Can you work these out from the model? Positions are in its coordinate system, mm. Give positions to 0.01 mm unless a question says otherwise; leave off trailing zeros. Loops run counter-clockwise (first coordinate to the right, second up) from the corner with the lowest first, then second, coordinate; pieces in that order, holes last. Notation, with made-up numbers: (19, 22.5) -> (28, 22.5) arc R32 ccw to (28, 49.5) -> close; hole circle Ø2 at (48, -8.5). An arc over 180 degrees is marked (long way). Return JSON: item names as keys, results as strings. Group by question number.
Q1. Suppose I cut it at D-D, the plane y = 13. Please give me the cut outline in (x, z), and give its area (3 significant figures).
Q2. Will these pins go through, and if not, where does the flat tip stop? pin 1 (6 mm diameter, centred on x = 0, y = 0, fed in from +Z); pin 2 (8 mm diameter, centred on x = 12, y = -8.5, fed in from +Z); pin 3 (2 mm diameter, centred on x = 12, z = 3, fed in from +Y).
Q3. Suppose I cut it at B-B, the plane y = 0. Please give me the cut outline in (x, z), and give its area (3 significant figures).
Q4. Suppose I cut it at A-A, the plane x = 0. Please give me the cut outline in (y, z).
Q5. I need wall thicknesses on line 1 along Y through (x, z) = (0, 0.5); line 2 along X through (y, z) = (-9, 1.3); line 3 along Z through (x, y) = (-2, 16). Which ranges of each line are inside material? Lowest first, please. Write a range as [from, to].
Q6. Suppose I cut it at C-C, the plane z = 2.9. Please give me the cut outline in (x, y), and give its area (3 significant figures).
```python
from build123d import *

# Parameters (mm, degrees)
EXTRUDE_1_DEPTH = 4
SKETCH_2_R      = 2.4
EXTRUDE_2_DEPTH = 1
FILLET_1_R      = 3


with BuildPart() as part:
    # 草圖1 → 填料-伸長1 (new body)
    with BuildSketch(Plane.XY):
        with BuildLine():
            Line((-7.867443673, 18.408334232), (-7.867443673, -19.856671438))
            Line((-7.867443673, -19.856671438), (-20, -19.856671438))
            Line((-20, -19.856671438), (0, -99.856671438))
            Line((0, -99.856671438), (20, -19.856671438))
            Line((20, -19.856671438), (7.867443673, -19.856671438))
            Line((7.867443673, -19.856671438), (7.867443673, 18.408334232))
            ThreePointArc((7.867443673, 18.408334232), (0, 23.981275915), (-7.867443673, 18.408334232))
        make_face()
        with BuildLine():
            ThreePointArc((-4.999271035, -4.154189345), (-6.5, 0), (-4.999271035, 4.154189345))
            Line((-4.999271035, 4.154189345), (-2.6, 17.94275172))
            ThreePointArc((-2.6, 17.94275172), (0, 20), (2.6, 17.94275172))
            Line((2.6, 17.94275172), (4.999271035, 4.154189345))
            ThreePointArc((4.999271035, 4.154189345), (6.5, 0), (4.999271035, -4.154189345))
            Line((4.999271035, -4.154189345), (2.6, -17.94275172))
            ThreePointArc((2.6, -17.94275172), (0, -20), (-2.6, -17.94275172))
            Line((-2.6, -17.94275172), (-4.999271035, -4.154189345))
        make_face(mode=Mode.SUBTRACT)
    extrude(amount=EXTRUDE_1_DEPTH)

    # 草圖2 → 填料-伸長2 (add)
    with BuildSketch(Plane.XY):
        with BuildLine():
            Line((-3.702325647, 20.172267208), (4.497563026, 20.172267208))
            ThreePointArc((4.497563026, 20.172267208), (6.068658829, 19.068237677), (7.032818959, 17.407629814))
            Line((7.032818959, 17.407629814), (7.032818959, -20.628324178))
            Line((7.032818959, -20.628324178), (-6.646673958, -20.628324178))
            Line((-6.646673958, -20.628324178), (-6.646673958, 17.471058727))
            ThreePointArc((-6.646673958, 17.471058727), (-5.621736824, 19.309156464), (-3.702325647, 20.172267208))
        make_face()
        Circle(SKETCH_2_R, mode=Mode.SUBTRACT)
    extrude(amount=EXTRUDE_2_DEPTH)

    # 圓角1
    fillet_1_edges = [part.edges().sort_by_distance(p)[0] for p in [
        (20, -19.856671438, 2),
        (0, -99.856671438, 2),
        (-20, -19.856671438, 2),
    ]]
    fillet(fillet_1_edges, radius=FILLET_1_R)


solid = part.part
```
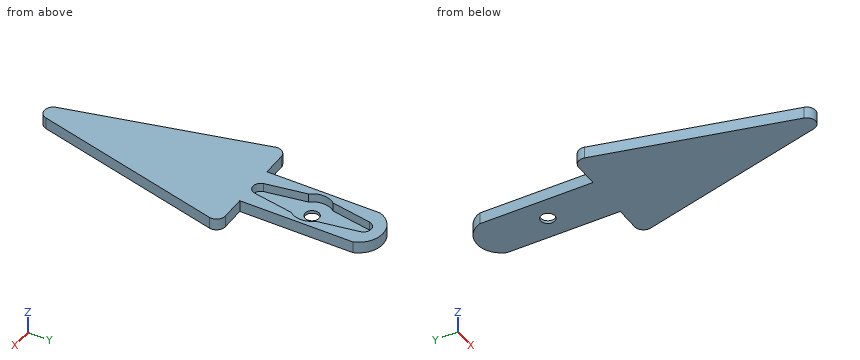
Ans:
{
 "1": {"outline": "(-7.87, 0) -> (7.87, 0) -> (7.87, 4) -> (3.46, 4) -> (3.46, 1) -> (-3.46, 1) -> (-3.46, 4) -> (-7.87, 4) -> close", "area": "42.2 mm^2"},
 "2": {"pin 1": "stops at z = 1", "pin 2": "passes through", "pin 3": "stops at y = -19.86"},
 "3": {"outline": "(-7.87, 0) -> (-2.4, 0) -> (-2.4, 1) -> (-6.5, 1) -> (-6.5, 4) -> (-7.87, 4) -> close; (2.4, 0) -> (7.87, 0) -> (7.87, 4) -> (6.5, 4) -> (6.5, 1) -> (2.4, 1) -> close", "area": "19.1 mm^2"},
 "4": {"outline": "(-90.49, 0) -> (-2.4, 0) -> (-2.4, 1) -> (-20, 1) -> (-20, 4) -> (-90.49, 4) -> close; (2.4, 0) -> (23.98, 0) -> (23.98, 4) -> (20, 4) -> (20, 1) -> (2.4, 1) -> close"},
 "5": {"line 1": "y = [-90.49, -2.4], [2.4, 23.98]", "line 2": "x = [-7.87, -4.16], [4.16, 7.87]", "line 3": "z = [0, 1]"},
 "6": {"outline": "(-19.07, -23.58) -> (-2.91, -88.21) arc R3 ccw to (2.91, -88.21) -> (19.07, -23.58) arc R3 ccw to (16.16, -19.86) -> (7.87, -19.86) -> (7.87, 18.41) arc R8.34 ccw to (-7.87, 18.41) -> (-7.87, -19.86) -> (-16.16, -19.86) arc R3 ccw to start; hole (-5, -4.15) -> (-2.6, -17.94) arc R2.67 ccw to (2.6, -17.94) -> (5, -4.15) arc R6.5 ccw to (5, 4.15) -> (2.6, 17.94) arc R2.67 ccw to (-2.6, 17.94) -> (-5, 4.15) arc R6.5 ccw to start", "area": "1,910 mm^2"}
}
